Check sheet for the modelled part. Datum: model origin and axes. Units: mm. A direction names the side the tool comes from. Coordinates: 2 decimals unless noted, no trailing zeros. Loops run counter-clockwise (first coordinate to the right, second up) from the corner with the lowest first, then second, coordinate; pieces in that order, holes last. Notation, with made-up numbers: (52, 35.25) -> (97, 35.25) arc R22 cw to (97, 51.25) -> close; hole circle Ø2 at (12, 85). An arc over 180 degrees is marked (long way). Use CSV: the item, a comma, the result in double quotes. Start each with the question number.
1. Release check for a two-part mould opening along Z. For faces 3 (the face through (15, 6, 0)), 4 (the face through (0.026, 6.338, 16.765)), 5 (the face through (-14.53, 6.34, -8.36)) record: pulls with the +Z half, pulls with the -Z half, needs draft (parallel to the pull), parting line crosses it, or undercut.
2. Gauge pin test, flat ends, axial feed: pin 1 (6 mm diameter, centred on x = 6, y = -32.5, fed in from +Z); pin 2 (2 mm diameter, centred on y = -29.5, z = 0.5, fed in from -X); pin 3 (3 mm diameter, centred on y = -37, z = -8, fed in from +X). Record the tip position at first contact, or that the pin passes through.
3. Thickness scan on L1, parallel to Y at x = 13.5, z = -3.5; L2, parallel to Z at x = 4.5, y = -26.5; L3, parallel to Z at x = 5, y = 9.5. Record the ranges inside material, lowest first.
4. Set-up check for faces 1 (the face through (-7, 0, -8)), 2 (the face through (-15, 6, 0)): record each of +Z, -Z, +X, -X, +Y, -Y from which the full face is reachable in a straight line by a thin tool's end or side.
5. Sectioned sample at D-D, the plane z = 13. Record the cut outline in (x, y), and give its area (3 significant figures).
6. Sectioned sample at A-A, the plane x = 0. Record the cut outline in (y, z) (3 decimals).
7. Sectioned sample at B-B, the plane z = 0. Record the cut outline in (x, y).
8. Sectioned sample at C-C, the plane y = -11. Record the cut outline in (x, z).
```python
from build123d import *

# Parameters (mm, degrees)
F2_R     = 25.1475
F3_DEPTH = 25


# Not quite as in the source:
# - a feature names something its author has since deleted; it is built from what else it names


with BuildPart() as f1:
    # F0 (on Right) → F1 (revolve)
    with BuildSketch(Plane.YZ):
        Polygon((0, 25.1475), (0, 10), (-43, 10), (-45, 8), (-45, 0), (12.5, 0), (12.5, 25.1475), align=None)
    revolve(axis=Axis((0, -16.25, 0), (0, -1, 0)))

    # F2 (on face) → F3 (cut)
    with BuildSketch(Plane(origin=(0, 12.5, 0), x_dir=(-1, 0, 0), z_dir=(0, 1, 0))):
        Circle(F2_R)
        with BuildLine():
            ThreePointArc((1.7954303246, -16.2839158944), (0, -16.765), (-1.7954303246, -16.2839158944))
            Line((-1.7954303246, -16.2839158944), (-13.2045696754, -9.6968462191))
            ThreePointArc((-13.2045696754, -9.6968462191), (-14.5189158944, -8.3825), (-15, -6.5870696754))
            Line((-15, -6.5870696754), (-15, 6.5870696754))
            ThreePointArc((-15, 6.5870696754), (-14.5189158944, 8.3825), (-13.2045696754, 9.6968462191))
            Line((-13.2045696754, 9.6968462191), (-1.7954303246, 16.2839158944))
            ThreePointArc((-1.7954303246, 16.2839158944), (0, 16.765), (1.7954303246, 16.2839158944))
            Line((1.7954303246, 16.2839158944), (13.2045696754, 9.6968462191))
            ThreePointArc((13.2045696754, 9.6968462191), (14.5189158944, 8.3825), (15, 6.5870696754))
            Line((15, 6.5870696754), (15, -6.5870696754))
            ThreePointArc((15, -6.5870696754), (14.5189158944, -8.3825), (13.2045696754, -9.6968462191))
            Line((13.2045696754, -9.6968462191), (1.7954303246, -16.2839158944))
        make_face(mode=Mode.SUBTRACT)
    extrude(amount=-F3_DEPTH, mode=Mode.SUBTRACT)


solid = f1.part
```
Completed:
1,face 3,"needs draft"
1,face 4,"pulls with the +Z half"
1,face 5,"pulls with the -Z half"
2,pin 1,"z = 9.54"
2,pin 2,"x = -10"
2,pin 3,"x = 7.6"
3,L1,"0 to 12.5"
3,L2,"-8.93 to 8.93"
3,L3,"-14.43 to 14.43"
4,face 1,"-Y"
4,face 2,"+Z, -Z, -X, +Y, -Y"
5,outline,"(-7.48, 0) -> (7.48, 0) -> (7.48, 12.5) -> (-7.48, 12.5) -> close"
5,area,"187 mm²"
6,outline,"(-45, -8) -> (-43, -10) -> (0, -10) -> (0, -16.765) -> (12.5, -16.765) -> (12.5, 16.765) -> (0, 16.765) -> (0, 10) -> (-43, 10) -> (-45, 8) -> close"
7,outline,"(-15, 0) -> (-10, 0) -> (-10, -43) -> (-8, -45) -> (8, -45) -> (10, -43) -> (10, 0) -> (15, 0) -> (15, 12.5) -> (-15, 12.5) -> close"
8,outline,"circle Ø20 at (0, 0)"
